Input: part model. Units: mm. Frame: model coordinates. Coordinates: 2 decimals unless noted, no trailing zeros. Loops run counter-clockwise (first coordinate to the right, second up) from the corner with the lowest first, then second, coordinate; pieces in that order, holes last. Notation, with made-up numbers: (82.25, -2) -> (129.25, -2) arc R7 ccw to (129.25, 7) -> close; hole circle Ø8 at (-0.75, 39.5). An arc over 180 degrees is marked (long way). Answer as a JSON object with one key per item and string values.
from build123d import *

# Parameters (mm, degrees)
F0_W         = 25.4
F0_H         = 25.4
F1_DEPTH     = 12.7
F5_D         = 14.2875
F5_ON_F3_D   = 14.2875
F5_ON_F2_D   = 14.2875
F6_T1_DEPTH  = 10.16
F6_T3_DEPTH  = 10.16
F6_T5_DEPTH  = 10.16
F6_S9_W      = 7.62
F6_S9_H      = 7.62
F6_T10_DEPTH = 7.62
F6_S15_W     = 7.62
F6_S15_H     = 7.62
F6_T16_DEPTH = 7.62
F6_S21_W     = 7.62
F6_S21_H     = 7.62
F6_T22_DEPTH = 7.62
F6_S27_W     = 7.62
F6_S27_H     = 7.62
F6_T28_DEPTH = 7.62
F6_S33_W     = 7.62
F6_S33_H     = 7.62
F6_T34_DEPTH = 7.62
F6_S39_W     = 7.62
F6_S39_H     = 7.62
F6_T40_DEPTH = 7.62
F6_S45_W     = 7.62
F6_S45_H     = 7.62
F6_T46_DEPTH = 7.62
F6_S51_W     = 7.62
F6_S51_H     = 7.62
F6_T52_DEPTH = 7.62


# Not quite as in the source:
# - a fillet or chamfer that OpenCascade refuses, or shapes differently, is made with other operations: its cross-section is extruded or revolved along the edge and cut away or added
# - a length typed as a fraction of an inch, garbled in the dataset ("3 / 203.2 mm" for 3/8 in), is restored


with BuildPart() as f1:
    # F0 (on Front) → F1 (new body, symmetric)
    with BuildSketch(Plane.XZ):
        Rectangle(F0_W, F0_H)
    extrude(amount=F1_DEPTH, both=True)

    # F5 (through all)
    with Locations(Plane.XY.offset(12.7)):
        with Locations((0, 0)):
            Hole(F5_D / 2)

    # F5 on F3 (through all)
    with Locations(Plane.XZ.offset(12.7)):
        with Locations((0, 0)):
            Hole(F5_ON_F3_D / 2)

    # F5 on F2 (through all)
    with Locations(Plane.YZ.offset(12.7)):
        with Locations((0, 0)):
            Hole(F5_ON_F2_D / 2)

    # F6: fillet of radius 7.62 on 12 edges, made by hand

    # F6_s2 → F6_t1 (cut)
    with BuildSketch(Plane.XZ.offset(-5.08)):
        with BuildLine():
            ThreePointArc((12.7, 5.08), (10.4681536726, 10.4681536726), (5.08, 12.7))
            Line((5.08, 12.7), (12.7, 12.7))
            Line((12.7, 12.7), (12.7, 5.08))
        make_face()
        with BuildLine():
            ThreePointArc((12.7, -5.08), (10.4681536726, -10.4681536726), (5.08, -12.7))
            Line((5.08, -12.7), (12.7, -12.7))
            Line((12.7, -12.7), (12.7, -5.08))
        make_face()
        with BuildLine():
            ThreePointArc((-5.08, 12.7), (-10.4681536726, 10.4681536726), (-12.7, 5.08))
            Line((-12.7, 5.08), (-12.7, 12.7))
            Line((-12.7, 12.7), (-5.08, 12.7))
        make_face()
        with BuildLine():
            ThreePointArc((-5.08, -12.7), (-10.4681536726, -10.4681536726), (-12.7, -5.08))
            Line((-12.7, -5.08), (-12.7, -12.7))
            Line((-12.7, -12.7), (-5.08, -12.7))
        make_face()
    extrude(amount=F6_T1_DEPTH, mode=Mode.SUBTRACT)

    # F6_s4 → F6_t3 (cut)
    with BuildSketch(Plane.XY.offset(-5.08)):
        with BuildLine():
            ThreePointArc((12.7, 5.08), (10.4681536726, 10.4681536726), (5.08, 12.7))
            Line((5.08, 12.7), (12.7, 12.7))
            Line((12.7, 12.7), (12.7, 5.08))
        make_face()
        with BuildLine():
            ThreePointArc((12.7, -5.08), (10.4681536726, -10.4681536726), (5.08, -12.7))
            Line((5.08, -12.7), (12.7, -12.7))
            Line((12.7, -12.7), (12.7, -5.08))
        make_face()
        with BuildLine():
            ThreePointArc((-5.08, -12.7), (-10.4681536726, -10.4681536726), (-12.7, -5.08))
            Line((-12.7, -5.08), (-12.7, -12.7))
            Line((-12.7, -12.7), (-5.08, -12.7))
        make_face()
        with BuildLine():
            ThreePointArc((-5.08, 12.7), (-10.4681536726, 10.4681536726), (-12.7, 5.08))
            Line((-12.7, 5.08), (-12.7, 12.7))
            Line((-12.7, 12.7), (-5.08, 12.7))
        make_face()
    extrude(amount=F6_T3_DEPTH, mode=Mode.SUBTRACT)

    # F6_s6 → F6_t5 (cut)
    with BuildSketch(Plane.YZ.offset(-5.08)):
        with BuildLine():
            ThreePointArc((-5.08, 12.7), (-10.4681536726, 10.4681536726), (-12.7, 5.08))
            Line((-12.7, 5.08), (-12.7, 12.7))
            Line((-12.7, 12.7), (-5.08, 12.7))
        make_face()
        with BuildLine():
            ThreePointArc((-5.08, -12.7), (-10.4681536726, -10.4681536726), (-12.7, -5.08))
            Line((-12.7, -5.08), (-12.7, -12.7))
            Line((-12.7, -12.7), (-5.08, -12.7))
        make_face()
        with BuildLine():
            ThreePointArc((12.7, 5.08), (10.4681536726, 10.4681536726), (5.08, 12.7))
            Line((5.08, 12.7), (12.7, 12.7))
            Line((12.7, 12.7), (12.7, 5.08))
        make_face()
        with BuildLine():
            ThreePointArc((12.7, -5.08), (10.4681536726, -10.4681536726), (5.08, -12.7))
            Line((5.08, -12.7), (12.7, -12.7))
            Line((12.7, -12.7), (12.7, -5.08))
        make_face()
    extrude(amount=F6_T5_DEPTH, mode=Mode.SUBTRACT)


with BuildPart() as f6_tool8:
    # F6_s9 → F6_t10 (new body)
    with BuildSketch(Plane.YZ.offset(5.08)):
        with Locations((8.89, 8.89)):
            Rectangle(F6_S9_W, F6_S9_H)
    extrude(amount=F6_T10_DEPTH)

    # F6_s11 → F6_t12 (revolve, cut)
    with BuildSketch(Plane(origin=(5.08, 5.08, 5.08), x_dir=(0, -0.7071067812, -0.7071067812), z_dir=(0, -0.7071067812, 0.7071067812))):
        with BuildLine():
            ThreePointArc((0, -7.62), (7.62, 0), (0, 7.62))
            Line((0, 7.62), (0, -7.62))
        make_face()
    revolve(axis=Axis((5.08, 5.08, 5.08), (1, 0, 0)), mode=Mode.SUBTRACT)


with BuildPart() as f1_1:
    add(f1.part)

    # F6_t7: cut F6_tool8
    add(f6_tool8.part, mode=Mode.SUBTRACT)


with BuildPart() as f6_tool14:
    # F6_s15 → F6_t16 (new body)
    with BuildSketch(Plane.YZ.offset(5.08)):
        with Locations((-8.89, 8.89)):
            Rectangle(F6_S15_W, F6_S15_H)
    extrude(amount=F6_T16_DEPTH)

    # F6_s17 → F6_t18 (revolve, cut)
    with BuildSketch(Plane(origin=(5.08, -5.08, 5.08), x_dir=(0, 0.7071067812, -0.7071067812), z_dir=(0, -0.7071067812, -0.7071067812))):
        with BuildLine():
            ThreePointArc((0, -7.62), (7.62, 0), (0, 7.62))
            Line((0, 7.62), (0, -7.62))
        make_face()
    revolve(axis=Axis((5.08, -5.08, 5.08), (1, 0, 0)), mode=Mode.SUBTRACT)


with BuildPart() as f1_2:
    add(f1_1.part)

    # F6_t13: cut F6_tool14
    add(f6_tool14.part, mode=Mode.SUBTRACT)


with BuildPart() as f6_tool20:
    # F6_s21 → F6_t22 (new body)
    with BuildSketch(Plane.YZ.offset(5.08)):
        with Locations((-8.89, -8.89)):
            Rectangle(F6_S21_W, F6_S21_H)
    extrude(amount=F6_T22_DEPTH)

    # F6_s23 → F6_t24 (revolve, cut)
    with BuildSketch(Plane(origin=(5.08, -5.08, -5.08), x_dir=(0, 0.7071067812, 0.7071067812), z_dir=(0, 0.7071067812, -0.7071067812))):
        with BuildLine():
            ThreePointArc((0, -7.62), (7.62, 0), (0, 7.62))
            Line((0, 7.62), (0, -7.62))
        make_face()
    revolve(axis=Axis((5.08, -5.08, -5.08), (1, 0, 0)), mode=Mode.SUBTRACT)


with BuildPart() as f1_3:
    add(f1_2.part)

    # F6_t19: cut F6_tool20
    add(f6_tool20.part, mode=Mode.SUBTRACT)


with BuildPart() as f6_tool26:
    # F6_s27 → F6_t28 (new body)
    with BuildSketch(Plane.YZ.offset(5.08)):
        with Locations((8.89, -8.89)):
            Rectangle(F6_S27_W, F6_S27_H)
    extrude(amount=F6_T28_DEPTH)

    # F6_s29 → F6_t30 (revolve, cut)
    with BuildSketch(Plane(origin=(5.08, 5.08, -5.08), x_dir=(0, -0.7071067812, 0.7071067812), z_dir=(0, 0.7071067812, 0.7071067812))):
        with BuildLine():
            ThreePointArc((0, -7.62), (7.62, 0), (0, 7.62))
            Line((0, 7.62), (0, -7.62))
        make_face()
    revolve(axis=Axis((5.08, 5.08, -5.08), (1, 0, 0)), mode=Mode.SUBTRACT)


with BuildPart() as f1_4:
    add(f1_3.part)

    # F6_t25: cut F6_tool26
    add(f6_tool26.part, mode=Mode.SUBTRACT)


with BuildPart() as f6_tool32:
    # F6_s33 → F6_t34 (new body)
    with BuildSketch(Plane.XY.offset(5.08)):
        with Locations((-8.89, -8.89)):
            Rectangle(F6_S33_W, F6_S33_H)
    extrude(amount=F6_T34_DEPTH)

    # F6_s35 → F6_t36 (revolve, cut)
    with BuildSketch(Plane(origin=(-5.08, -5.08, 5.08), x_dir=(0.7071067812, 0.7071067812, 0), z_dir=(0.7071067812, -0.7071067812, 0))):
        with BuildLine():
            ThreePointArc((0, -7.62), (7.62, 0), (0, 7.62))
            Line((0, 7.62), (0, -7.62))
        make_face()
    revolve(axis=Axis((-5.08, -5.08, 5.08), (0, 0, 1)), mode=Mode.SUBTRACT)


with BuildPart() as f1_5:
    add(f1_4.part)

    # F6_t31: cut F6_tool32
    add(f6_tool32.part, mode=Mode.SUBTRACT)


with BuildPart() as f6_tool38:
    # F6_s39 → F6_t40 (new body)
    with BuildSketch(Plane.XY.offset(-5.08)):
        with Locations((-8.89, -8.89)):
            Rectangle(F6_S39_W, F6_S39_H)
    extrude(amount=-F6_T40_DEPTH)

    # F6_s41 → F6_t42 (revolve, cut)
    with BuildSketch(Plane(origin=(-5.08, -5.08, -5.08), x_dir=(0.7071067812, 0.7071067812, 0), z_dir=(-0.7071067812, 0.7071067812, 0))):
        with BuildLine():
            ThreePointArc((0, -7.62), (7.62, 0), (0, 7.62))
            Line((0, 7.62), (0, -7.62))
        make_face()
    revolve(axis=Axis((-5.08, -5.08, -5.08), (0, 0, -1)), mode=Mode.SUBTRACT)


with BuildPart() as f1_6:
    add(f1_5.part)

    # F6_t37: cut F6_tool38
    add(f6_tool38.part, mode=Mode.SUBTRACT)


with BuildPart() as f6_tool44:
    # F6_s45 → F6_t46 (new body)
    with BuildSketch(Plane.XZ.offset(-5.08)):
        with Locations((-8.89, 8.89)):
            Rectangle(F6_S45_W, F6_S45_H)
    extrude(amount=-F6_T46_DEPTH)

    # F6_s47 → F6_t48 (revolve, cut)
    with BuildSketch(Plane(origin=(-5.08, 5.08, 5.08), x_dir=(0.7071067812, 0, -0.7071067812), z_dir=(0.7071067812, 0, 0.7071067812))):
        with BuildLine():
            ThreePointArc((0, -7.62), (7.62, 0), (0, 7.62))
            Line((0, 7.62), (0, -7.62))
        make_face()
    revolve(axis=Axis((-5.08, 5.08, 5.08), (0, 1, 0)), mode=Mode.SUBTRACT)


with BuildPart() as f1_7:
    add(f1_6.part)

    # F6_t43: cut F6_tool44
    add(f6_tool44.part, mode=Mode.SUBTRACT)


with BuildPart() as f6_tool50:
    # F6_s51 → F6_t52 (new body)
    with BuildSketch(Plane.XZ.offset(-5.08)):
        with Locations((-8.89, -8.89)):
            Rectangle(F6_S51_W, F6_S51_H)
    extrude(amount=-F6_T52_DEPTH)

    # F6_s53 → F6_t54 (revolve, cut)
    with BuildSketch(Plane(origin=(-5.08, 5.08, -5.08), x_dir=(0.7071067812, 0, 0.7071067812), z_dir=(-0.7071067812, 0, 0.7071067812))):
        with BuildLine():
            ThreePointArc((0, -7.62), (7.62, 0), (0, 7.62))
            Line((0, 7.62), (0, -7.62))
        make_face()
    revolve(axis=Axis((-5.08, 5.08, -5.08), (0, 1, 0)), mode=Mode.SUBTRACT)


with BuildPart() as f1_8:
    add(f1_7.part)

    # F6_t49: cut F6_tool50
    add(f6_tool50.part, mode=Mode.SUBTRACT)


solid = f1_8.part
1. Section query D-D (x = 10.25). Return loops of the section in (y, z).
Reply:
{"outline": "(-10.68, -5.08) arc R5.6 ccw to (-5.08, -10.68) -> (5.08, -10.68) arc R5.6 ccw to (10.68, -5.08) -> (10.68, 5.08) arc R5.6 ccw to (5.08, 10.68) -> (-5.08, 10.68) arc R5.6 ccw to (-10.68, 5.08) -> close; hole circle Ø14.29 at (0, 0)"}
2. Pin query (flat end, axial travel): P1, Ø3, axis at x = 1.5, z = 5.5, coming from the +Y side; P2, Ø1, axis at y = 7.5, z = -8, coming from the -X side; P3, Ø1, axis at x = -6, z = 3, coming from the +Y side. Return the tip coordinate at first contact, or that it passes through.
Reply:
{"P1": "stops at y = 12.51", "P2": "stops at x = -11.95", "P3": "stops at y = 12.61"}
3. Section query C-C (x = -1.5). Return loops of the section in (y, z).
Reply:
{"outline": "(-12.46, -6.98) arc R7.62 ccw to (-6.98, -12.46) -> (-6.98, -6.98) -> close; (-12.46, 6.98) -> (-6.98, 6.98) -> (-6.98, 12.46) arc R7.62 ccw to start; (6.98, -12.46) arc R7.62 ccw to (12.46, -6.98) -> (6.98, -6.98) -> close; (6.98, 6.98) -> (12.46, 6.98) arc R7.62 ccw to (6.98, 12.46) -> close"}
4. Mould query, pull axis X, two halves, no side actions, for faces 1 (the face through (-10.409, 10.527, -0.071)), 2 (the face through (10.527, 0.071, 10.409)), 3 (the face through (0.93, 7.083, 9.672)). Classes: pulls with the +X half, pulls with the -X half, needs draft (parallel to the pull), parting line crosses it, or undercut.
Reply:
{"face 1": "pulls with the -X half", "face 2": "pulls with the +X half", "face 3": "undercut"}
5. Section query A-A (z = 6.75). Return loops of the section in (x, y), plus the area to 3 significant figures.
Reply:
{"outline": "(-12.51, -5.08) arc R7.43 ccw to (-5.08, -12.51) -> (-2.34, -12.51) -> (-2.34, -6.75) arc R7.14 cw to (-6.75, -2.34) -> (-12.51, -2.34) -> close; (-12.51, 2.34) -> (-6.75, 2.34) arc R7.14 cw to (-2.34, 6.75) -> (-2.34, 12.51) -> (-5.08, 12.51) arc R7.43 ccw to (-12.51, 5.08) -> close; (2.34, -12.51) -> (5.08, -12.51) arc R7.43 ccw to (12.51, -5.08) -> (12.51, -2.34) -> (6.75, -2.34) arc R7.14 cw to (2.34, -6.75) -> close; (2.34, 6.75) arc R7.14 cw to (6.75, 2.34) -> (12.51, 2.34) -> (12.51, 5.08) arc R7.43 ccw to (5.08, 12.51) -> (2.34, 12.51) -> close", "area": "316 mm2"}
6. Section query B-B (y = -5.75). Return loops of the section in (x, z).
Reply:
{"outline": "(-12.67, -5.08) arc R7.59 ccw to (-5.08, -12.67) -> (-4.24, -12.67) -> (-4.24, -5.75) arc R7.14 cw to (-5.75, -4.24) -> (-12.67, -4.24) -> close; (-12.67, 4.24) -> (-5.75, 4.24) arc R7.14 cw to (-4.24, 5.75) -> (-4.24, 12.67) -> (-5.08, 12.67) arc R7.59 ccw to (-12.67, 5.08) -> close; (4.24, -12.67) -> (5.08, -12.67) arc R7.59 ccw to (12.67, -5.08) -> (12.67, -4.24) -> (5.75, -4.24) arc R7.14 cw to (4.24, -5.75) -> close; (4.24, 5.75) arc R7.14 cw to (5.75, 4.24) -> (12.67, 4.24) -> (12.67, 5.08) arc R7.59 ccw to (5.08, 12.67) -> (4.24, 12.67) -> close"}
7. Line query: line 1 along Y through (x, z) = (-9.5, 3); line 2 along X through (y, z) = (-4.5, 8); line 3 along Z through (x, y) = (-3.25, 8). Output: solid intervals per line, ascending.
Reply:
{"line 1": "y = -11.29 to -6.48, 6.48 to 11.29", "line 2": "x = -12.12 to -5.55, 5.55 to 12.12", "line 3": "z = -12.12 to -6.36, 6.36 to 12.12"}
